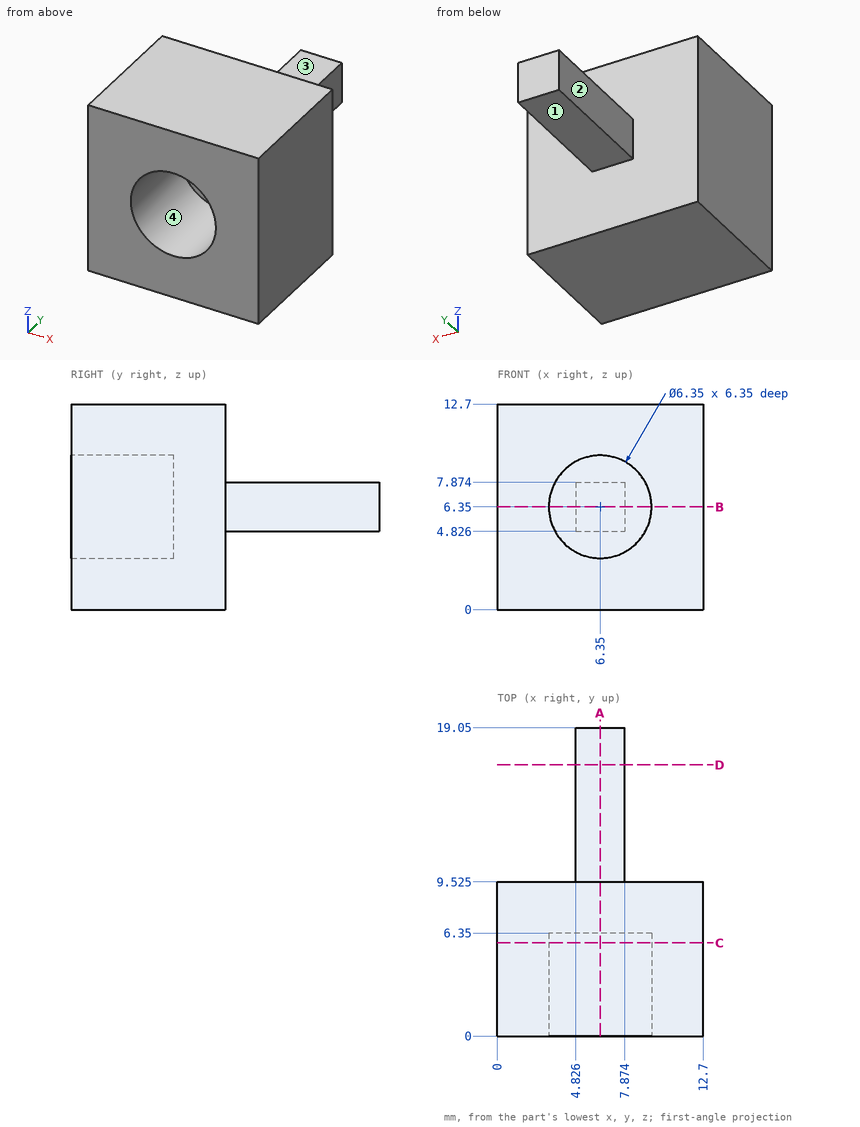
Study the drawing (mm; zero at the part's minimum x, y, z) and answer. Coordinates: 2 decimals unless noted, no trailing zeros. Write each loop counter-clockwise with the first axis right and the second up, starting at its lowest first coordinate (ties: lowest second). Pieces come first, ordered by that corner, then holes. Notation, with made-up numbers: (89, -8) - (130, -8) arc R11 ccw to (130, 1) - close; hole circle Ø5 at (-16, 18). An arc over 180 degrees is marked (long way). Answer as a JSON object with one key per item and string values. Group by question number.
1. Consider L1, parallel to X at y = 4.5, z = 6.35 (3 decimals); L2, parallel to Y at x = 12, z = 10 (3 decimals); L3, parallel to Z at x = 7.5, y = 15. Determine where each line is inside the solid, lowest interval first. Write a range as [from, to].
2. Each of these flat-tipped pins is pushed along its axis until it touches: P1, Ø6, axis at x = 3.5, z = 10.5, coming from the -Y side; P2, Ø3, axis at x = 6.5, y = 14, coming from the +Z side; P3, Ø0.9, axis at y = 13, z = 7, coming from the -X side; P4, Ø0.9, axis at y = 14, z = 7, coming from the +X side. Where does it stop, or does it pass through?
3. The mould has two halves that part along Z. Classify the marked faces 1, 2, 3 and 4: +Z half, -Z half, draft (parallel to the pull), parting line (faces both ways), or undercut.
4. A cutting plane is placed at C-C (y = 5.75). Determine the outline of the cut face in (x, z) (3 decimals), plus the area to 3 significant figures.
5. A cutting plane is placed at B-B (z = 6.35). Determine the outline of the cut face in (x, y) (3 decimals).
6. A cutting plane is placed at D-D (y = 16.75). Determine the outline of the cut face in (x, z), plus the area to 3 significant figures.
7. A cutting plane is placed at A-A (x = 6.35). Determine the outline of the cut face in (y, z) (3 decimals).
Worked out:
{
 "1": {"L1": "x = [0, 3.175], [9.525, 12.7]", "L2": "y = [0, 9.525]", "L3": "z = [4.83, 7.87]"},
 "2": {"P1": "stops at y = 0", "P2": "stops at z = 7.87", "P3": "stops at x = 4.83", "P4": "stops at x = 7.87"},
 "3": {"face 1": "-Z half", "face 2": "draft", "face 3": "+Z half", "face 4": "undercut"},
 "4": {"outline": "(0, 0) - (12.7, 0) - (12.7, 12.7) - (0, 12.7) - close; hole circle Ø6.35 at (6.35, 6.35)", "area": "130 mm²"},
 "5": {"outline": "(0, 0) - (3.175, 0) - (3.175, 6.35) - (9.525, 6.35) - (9.525, 0) - (12.7, 0) - (12.7, 9.525) - (7.874, 9.525) - (7.874, 19.05) - (4.826, 19.05) - (4.826, 9.525) - (0, 9.525) - close"},
 "6": {"outline": "(4.83, 4.83) - (7.87, 4.83) - (7.87, 7.87) - (4.83, 7.87) - close", "area": "9.29 mm²"},
 "7": {"outline": "(0, 0) - (9.525, 0) - (9.525, 4.826) - (19.05, 4.826) - (19.05, 7.874) - (9.525, 7.874) - (9.525, 12.7) - (0, 12.7) - (0, 9.525) - (6.35, 9.525) - (6.35, 3.175) - (0, 3.175) - close"}
}
